from build123d import *

# Parameters (mm, degrees)
SKETCH1_R                      = 79.375
BOSS_EXTRUDE1_DEPTH            = 3.175
SKETCH5_R                      = 10.4
CUT_EXTRUDE1_DEPTH             = 2.5
SKETCH6_R                      = 5
CUT_EXTRUDE2_DEPTH             = 113.432663181
CBORE_FOR_M2_SHCS1_D           = 2.2
CBORE_FOR_M2_SHCS1_DEPTH       = 6
CBORE_FOR_M2_SHCS1_CBORE_D     = 4.4
CBORE_FOR_M2_SHCS1_CBORE_DEPTH = 2
CBORE_FOR_M2_SHCS1_TIP         = 0.660946681
M4_CLEARANCE_HOLE1_D           = 4.5
M5_CLEARANCE_HOLE1_D           = 5.5


with BuildPart() as part:
    # Sketch1 → Boss-Extrude1 (new, symmetric)
    with BuildSketch(Plane(origin=(0, 0, 0), x_dir=(1, 0, 0), z_dir=(0, 1, 0))):
        with Locations(Location((0, 0, 0), (0, 0, 270))):
            Circle(SKETCH1_R)
    extrude(amount=BOSS_EXTRUDE1_DEPTH, both=True)

    # Sketch5 → Cut-Extrude1 (cut)
    with BuildSketch(Plane(origin=(0, 3.175, 0), x_dir=(1, 0, 0), z_dir=(0, 1, 0))):
        with Locations(Location((0, 0, 0), (0, 0, 270))):
            Circle(SKETCH5_R)
    extrude(amount=-CUT_EXTRUDE1_DEPTH, mode=Mode.SUBTRACT)

    # Sketch6 → Cut-Extrude2 (cut, through all)
    with BuildSketch(Plane(origin=(0, 3.175, 0), x_dir=(1, 0, 0), z_dir=(0, 1, 0))):
        with Locations(Location((0, 0, 0), (0, 0, 270))):
            Circle(SKETCH6_R)
    extrude(amount=-CUT_EXTRUDE2_DEPTH, mode=Mode.SUBTRACT)

    # CBORE for M2 SHCS1
    with Locations(Plane(origin=(0, 0.675, 0), x_dir=(1, 0, 0), z_dir=(0, 1, 0))):
        with Locations((-5.65685425, 5.65685425), (0, 8), (5.65685425, 5.65685425), (8, 0), (5.65685425, -5.65685425), (0, -8), (-5.65685425, -5.65685425), (-8, 0)):
            CounterBoreHole(CBORE_FOR_M2_SHCS1_D / 2, CBORE_FOR_M2_SHCS1_CBORE_D / 2, CBORE_FOR_M2_SHCS1_CBORE_DEPTH, depth=CBORE_FOR_M2_SHCS1_DEPTH)
            with Locations((0, 0, -(CBORE_FOR_M2_SHCS1_DEPTH + CBORE_FOR_M2_SHCS1_TIP / 2))):  # 118° drill point
                Cone(0, CBORE_FOR_M2_SHCS1_D / 2, CBORE_FOR_M2_SHCS1_TIP, mode=Mode.SUBTRACT)

    # M4 Clearance Hole1 (through all)
    with Locations(Plane(origin=(0, 3.175, 0), x_dir=(1, 0, 0), z_dir=(0, 1, 0))):
        with Locations((19.05, -44.388212048), (-19.05, -44.388212048)):
            Hole(M4_CLEARANCE_HOLE1_D / 2)

    # M5 Clearance Hole1 (through all)
    with Locations(Plane(origin=(0, 3.175, 0), x_dir=(1, 0, 0), z_dir=(0, 1, 0))):
        with Locations((-33.6688086, 31.567387952), (-14.6188086, 31.567387952), (4.4311914, 31.567387952), (-15.875, -19.249706448), (15.875, -19.249706448)):
            Hole(M5_CLEARANCE_HOLE1_D / 2)


solid = part.part
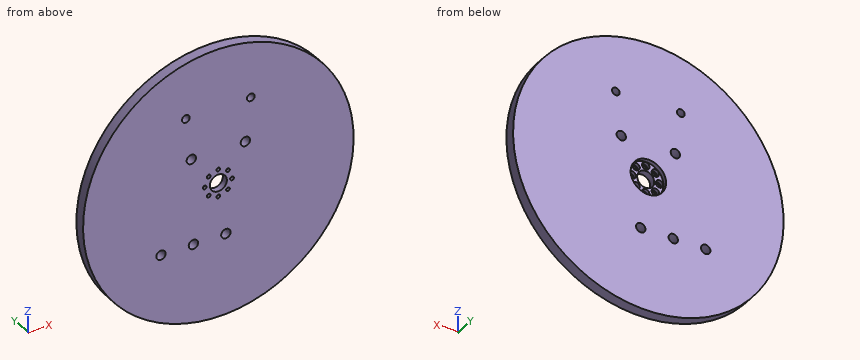
CAD build for the part. Positions are in the model's coordinates, mm. Round coordinates to 2 decimals unless told otherwise and drop trailing zeros. Order: outer loops, then holes, each group sorted by start corner. A loop starts at its lowest first (then second) coordinate and runs counter-clockwise, first axis right, second up. Notation, with made-up numbers: (77, 76) -> (88, 76) arc R14 cw to (88, 91) -> close; hole circle Ø6 at (31, 9.25). An arc over 180 degrees is marked (long way). Write each question's results on one line, items separated by ' | '.
1. Wall check: line 1 along X through (y, z) = (1, 43); line 2 along Z through (x, y) = (3, -2); line 3 along X through (y, z) = (0.75, 43.5). Give the ranges that are in metal, low to high. Write a range as [from, to].
Findings below:
line 1: x = [-66.72, -20.82], [-17.28, 17.28], [20.82, 66.72] | line 2: z = [-79.32, -33.92], [-29.22, -4], [4, 79.32] | line 3: x = [-66.39, -21.12], [-16.98, 16.98], [21.12, 66.39]
2. Cut at B-B (x = 29). Give the cut face in (y, z) (3 decimals), plus the area to 3 significant figures.
Findings below:
outline: (-3.175, -73.888) -> (3.175, -73.888) -> (3.175, 73.888) -> (-3.175, 73.888) -> close | area: 938 mm²
3. Cut at C-C (z = 61.5). Give the cut face in (x, y) (3 decimals).
Findings below:
outline: (-50.181, -3.175) -> (50.181, -3.175) -> (50.181, 3.175) -> (-50.181, 3.175) -> close
4. Flat gauge pins, fed straight in: P1, Ø3.5, axis at x = 0, z = -8, coming from the -Y side (3 decimals); P2, Ø2, axis at x = -5.66, z = -5.66, coming from the -Y side; P3, Ø1.3, axis at x = 6.5, z = 5, coming from the +Y side (3 decimals); P4, Ø2, axis at y = -0.5, z = 6.5, coming from the +X side. Where does each tip first touch, or does it go through?
Findings below:
P1: stops at y = -3.175 | P2: passes through | P3: stops at y = -1.325 | P4: stops at x = 79.18
5. Cut at A-A (y = 2). Count the separate pieces of the cut face and the enclosed holes in it, plus the area to 3 significant figures.
Findings below:
separate pieces: 1 | enclosed holes: 8 | area: 19,300 mm²
